For this review, use the dimensioned drawing (mm, ordinates from the lowest corner) and the shaded views. Coordinates: 2 decimals unless noted, no trailing zeros. One line per item, written item: value. Start each with the question number.
1. Insertion check: P1, Ø4, axis at x = 20.84, y = 25.04, coming from the +Z side (1 decimal); P2, Ø3.5, axis at x = 43.22, y = 18.73, coming from the -Z side. Each pin has a flat end and moves straight along its axis. Give the tip position at first contact, or say it passes through.
2. To check wall thickness, follow line 1 (Y direction, x = 20, z = 3.35); line 2 (Y direction, x = 41, z = 4.5) (1 decimal); line 3 (X direction, y = 25.5, z = 0.6). State the ranges of each line that lie inside material, in increasing order.
3. We need section A-A, the plane z = 1.7. Count the separate pieces of the cut face and the enclosed holes in it, then the cut area to 3 significant figures.
4. Mouldability with a two-part tool opening along Y and no side actions: class the marked faces 1 and 2 as +Y half, -Y half, draft (parallel to the pull), parting line (faces both ways), or undercut.
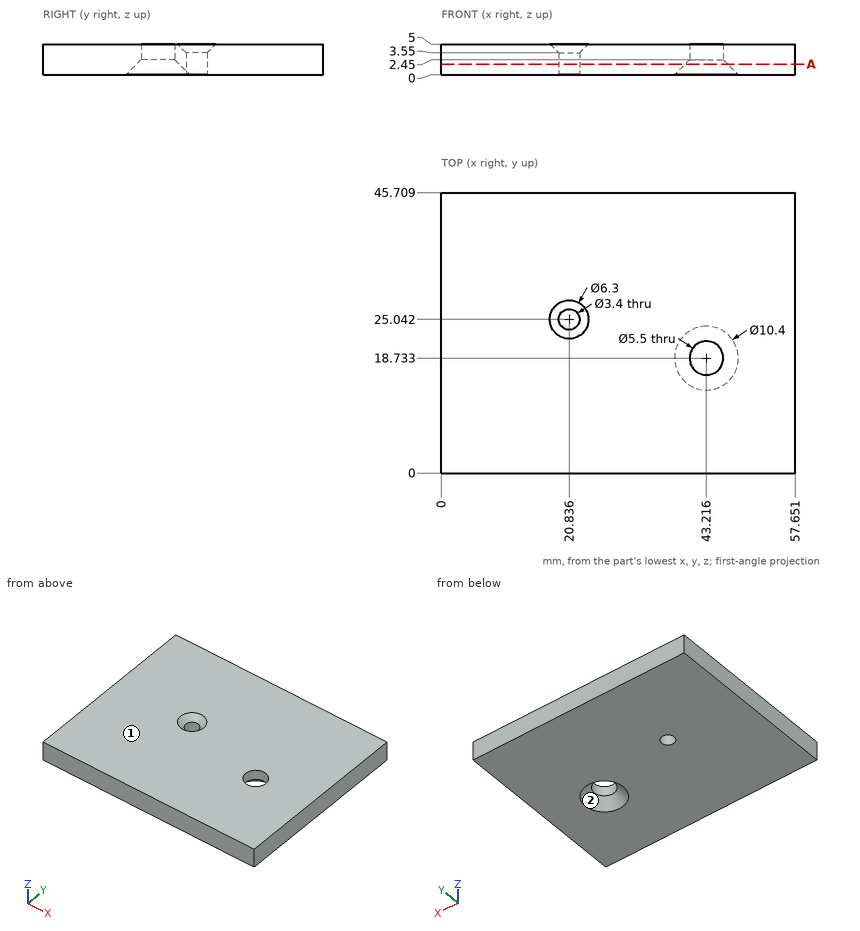
Findings below:
1. P1: z = 3.9
1. P2: through
2. line 1: 0 to 23.56, 26.52 to 45.71
2. line 2: 0 to 17.1, 20.4 to 45.7
2. line 3: 0 to 19.2, 22.47 to 57.65
3. separate pieces: 1
3. enclosed holes: 2
3. area: 2,590 mm2
4. face 1: draft
4. face 2: undercut
